The drawing under review shows one solid part. Ordinate dimensions are in mm from its lowest x, y, z. Coordinates: 2 decimals unless noted, no trailing zeros. Loops run counter-clockwise (first coordinate to the right, second up) from the corner with the lowest first, then second, coordinate; pieces in that order, holes last. Notation, with made-up numbers: M 35,29 L 76,29 A31 cw 76,68 Z; hole C -16.5,81.25 d5. An arc over 180 degrees is marked long. Use one line per item in the form item = value.
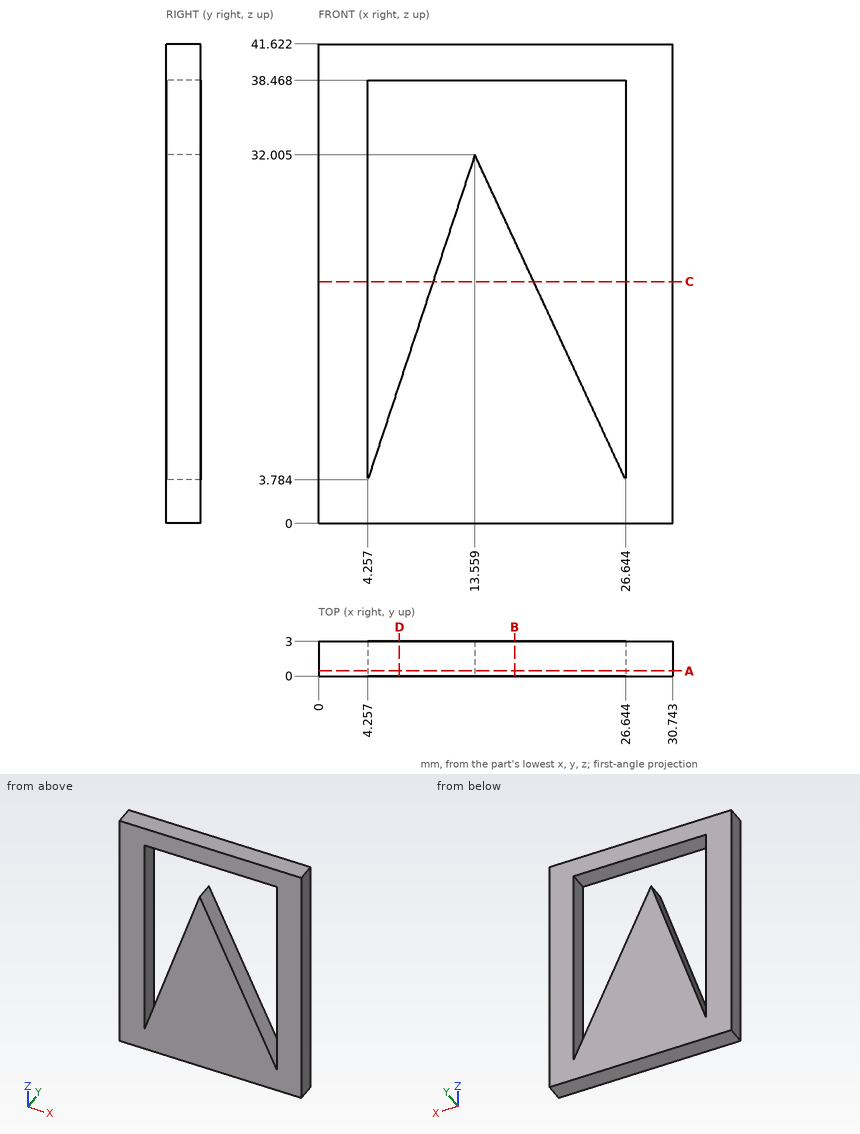
1. Consider section D-D on x = 7. Write out the cut boundary in (y, z).
Computed values:
outline = M 0,0 L 3,0 L 3,12.11 L 0,12.11 Z; M 0,38.47 L 3,38.47 L 3,41.62 L 0,41.62 Z
2. Consider section A-A on y = 0.45. Write out the cut boundary in (x, z) (1 decimal), plus the area to 3 significant figures.
Computed values:
outline = M 0,0 L 30.7,0 L 30.7,41.6 L 0,41.6 Z; hole M 4.3,3.8 L 13.6,32 L 26.6,3.8 L 26.6,38.5 L 4.3,38.5 Z
area = 819 mm2
3. Consider section C-C on z = 21. Write out the cut boundary in (x, y) (1 decimal).
Computed values:
outline = M 0,0 L 4.3,0 L 4.3,3 L 0,3 Z; M 9.9,0 L 18.7,0 L 18.7,3 L 9.9,3 Z; M 26.6,0 L 30.7,0 L 30.7,3 L 26.6,3 Z
4. Consider section B-B on x = 17. Write out the cut boundary in (y, z).
Computed values:
outline = M 0,0 L 3,0 L 3,24.58 L 0,24.58 Z; M 0,38.47 L 3,38.47 L 3,41.62 L 0,41.62 Z
5. For pin 1 Ø4 at (x, z) = (15.5, 33) entering from +Y, flat-tipped, find the tip position at first contact; note if it passes through.
Computed values:
pin_1 = through
6. Wall thickness on line 1 along X through (y, z) = (0.85, 18) (1 decimal); line 2 along X through (y, z) = (0.4, 9) (1 decimal); line 3 along X through (y, z) = (0.9, 34.5) (1 decimal): over which ranges is each line inside the solid? List them lowest first. Write a range as from..to.
Computed values:
line_1 = 0..4.3, 8.9..20.1, 26.6..30.7
line_2 = 0..4.3, 6..24.2, 26.6..30.7
line_3 = 0..4.3, 26.6..30.7
